Source: CAD feature listing. Evaluate the final solid. Frame: model axes, mm. A direction names the side the tool comes from. Coordinates: 2 decimals unless noted, no trailing zeros. Order: outer loops, then holes, each group sorted by start corner. A loop starts at its lowest first (then second) coordinate and runs counter-clockwise, first axis right, second up. Notation, with made-up numbers: (34, 46.5) - (84, 46.5) arc R24 ccw to (84, 59.5) - close; hole circle Ø6 at (52.5, 2.5). An arc over 180 degrees is marked (long way). One line per question, with ' | ' between items.
from build123d import *

# Parameters (mm, degrees)
EXTRUDE1_DEPTH     = 247.65
SKETCH2_W          = 34.925
SKETCH2_H          = 9.525
CUT_EXTRUDE1_DEPTH = 12.7
SKETCH3_W          = 2.38125
SKETCH3_H          = 22.225
SKETCH3_H_2        = 28.575
EXTRUDE2_DEPTH     = 15.875
FILLET1_R          = 1.5875
SKETCH4_W          = 4.7625
SKETCH4_H          = 25.4
CUT_EXTRUDE2_DEPTH = 2.38125
CUT_EXTRUDE3_DEPTH = 6.35
SKETCH6_R          = 3.96875
CUT_EXTRUDE4_DEPTH = 2.38125


with BuildPart() as part:
    # Sketch1 → Extrude1 (new, symmetric)
    with BuildSketch(Plane.XY):
        with BuildLine():
            Line((0, 46.0375), (0, 0))
            Line((0, 0), (2.38125, 0))
            Line((2.38125, 0), (2.38125, 46.0375))
            ThreePointArc((2.38125, 46.0375), (3.078701977, 47.721298023), (4.7625, 48.41875))
            Line((4.7625, 48.41875), (26.9875, 48.41875))
            ThreePointArc((26.9875, 48.41875), (30.355096045, 49.813653955), (31.75, 53.18125))
            Line((31.75, 53.18125), (31.75, 61.11875))
            Line((31.75, 61.11875), (29.36875, 61.11875))
            Line((29.36875, 61.11875), (29.36875, 53.18125))
            ThreePointArc((29.36875, 53.18125), (28.671298023, 51.497451977), (26.9875, 50.8))
            Line((26.9875, 50.8), (4.7625, 50.8))
            ThreePointArc((4.7625, 50.8), (1.394903955, 49.405096045), (0, 46.0375))
        make_face()
    extrude(amount=EXTRUDE1_DEPTH, both=True)

    # Sketch2 → Cut-Extrude1 (cut)
    with BuildSketch(Plane.ZY):
        with Locations((-139.7, 46.0375)):
            Rectangle(SKETCH2_W, SKETCH2_H)
        with Locations((139.7, 46.0375)):
            Rectangle(SKETCH2_W, SKETCH2_H)
    extrude(amount=-CUT_EXTRUDE1_DEPTH, mode=Mode.SUBTRACT)

    # Sketch3 → Extrude2 (add)
    with BuildSketch(Plane(origin=(0, 41.275, 0), x_dir=(1, 0, 0), z_dir=(0, 1, 0))):
        with Locations((1.190625, 142.875)):
            Rectangle(SKETCH3_W, SKETCH3_H)
        with Locations((1.190625, -139.7)):
            Rectangle(SKETCH3_W, SKETCH3_H_2)
    extrude(amount=EXTRUDE2_DEPTH)

    # Fillet1
    fillet1_edges = [part.edges().sort_by_distance(p)[0] for p in [
        (1.190625, 41.275, 125.4125),
        (1.190625, 41.275, 153.9875),
        (1.190625, 41.275, -157.1625),
        (1.190625, 41.275, 157.1625),
        (1.190625, 41.275, 122.2375),
        (1.190625, 41.275, -153.9875),
        (1.190625, 41.275, -131.7625),
    ]]
    fillet(fillet1_edges, radius=FILLET1_R - 0.0001)  # a hair under: the kernel refuses the full size

    # Sketch4 → Cut-Extrude2 (cut)
    with BuildSketch(Plane(origin=(0, 50.8, 0), x_dir=(1, 0, 0), z_dir=(0, 1, 0))):
        with Locations((13.49375, 207.9625)):
            Rectangle(SKETCH4_W, SKETCH4_H)
        with Locations((11.90625, -193.675)):
            Rectangle(SKETCH4_W, SKETCH4_H)
    extrude(amount=-CUT_EXTRUDE2_DEPTH, mode=Mode.SUBTRACT)

    # Sketch5 → Cut-Extrude3 (cut)
    with BuildSketch(Plane(origin=(31.75, 0, 0), x_dir=(0, 0, -1), z_dir=(1, 0, 0))):
        Polygon((195.2625, 61.11875), (220.6625, 61.11875), (218.28125, 50.8), (218.28125, 48.41875), (197.64375, 48.41875), (197.64375, 50.8), align=None)
        Polygon((-180.975, 61.11875), (-206.375, 61.11875), (-203.99375, 50.8), (-203.99375, 48.41875), (-183.35625, 48.41875), (-183.35625, 50.8), align=None)
    extrude(amount=-CUT_EXTRUDE3_DEPTH, mode=Mode.SUBTRACT)

    # Sketch6 → Cut-Extrude4 (cut)
    with BuildSketch(Plane.ZY):
        with Locations((0, 22.225)):
            Circle(SKETCH6_R)
    extrude(amount=-CUT_EXTRUDE4_DEPTH, mode=Mode.SUBTRACT)


solid = part.part
(1) Cut plane C-C (y = 35). Return the cut outline in (x, z).
Taken from the geometry:
outline: (0, -247.65) - (2.38, -247.65) - (2.38, 247.65) - (0, 247.65) - close
(2) Pull-direction query (Y, two-part tool) for faces 1 (the cylindrical face through (1.17, 18.35, -0.86)), 2 (the flat face through (16, 50.8, 3)), 3 (the flat face through (31.75, 57, -4)), 4 (the flat face through (16, 48.419, 3)); classes: pulls with the +Y half, pulls with the -Y half, needs draft (parallel to the pull), parting line crosses it, or undercut.
Taken from the geometry:
face 1: undercut | face 2: pulls with the +Y half | face 3: needs draft | face 4: pulls with the -Y half
(3) Material intervals for L1, parallel to Y at x = 0.65, z = 0; L2, parallel to Y at x = 20, z = 59; L3, parallel to X at y = 32, z = 67.5, sorted ascending. Write a range as from..to.
Taken from the geometry:
L1: y = 0..18.26, 26.19..48.44 | L2: y = 48.42..50.8 | L3: x = 0..2.38
(4) Cut plane B-B (x = 20). Return the cut outline in (y, z), and give its area (3 significant figures).
Taken from the geometry:
outline: (48.42, -247.65) - (50.8, -247.65) - (50.8, 247.65) - (48.42, 247.65) - close | area: 1,180 mm²
(5) Pin query (flat end, axial travel): P1, Ø2.5, axis at x = 1.5, y = 53, coming from the -Z side; P2, Ø1.9, axis at y = 50, z = 200, coming from the -X side; P3, Ø8.5, axis at x = 3.5, y = 46.5, coming from the +Z side; P4, Ø2.5, axis at y = 49.5, z = -203, coming from the +X side. Return the tip coordinate at first contact, or that it passes through.
Taken from the geometry:
P1: stops at z = -153.99 | P2: stops at x = 1.07 | P3: stops at z = 247.65 | P4: stops at x = 25.4
(6) Set-up query: faces 5 (the flat face through (31.75, 57, 226)), 6 (the flat face through (29.369, 57, -233)), 7 (the flat face through (3, 48, -122.237)). Return all of +Z, -Z, +X, -X, +Y, -Y with unobstructed straight access to the full face (end or side cutting, diameter ignored); none if empty.
Taken from the geometry:
face 5: +Z, -Z, +X, +Y, -Y | face 6: +Z, -Z, -X, +Y | face 7: -X, +Y
